Work out the finished part from the listing and answer in its coordinate system (mm). Coordinates: 2 decimals unless noted, no trailing zeros. Order: outer loops, then holes, each group sorted by start corner. A loop starts at its lowest first (then second) coordinate and runs counter-clockwise, first axis right, second up. Notation, with made-up numbers: (73, 84.5) -> (89, 84.5) arc R11 cw to (89, 102.5) -> close; hole circle Ø9 at (78, 89). An arc over 180 degrees is marked (long way). Write item = value, one per line. Start each with the question number.
Q1. Flat-ended cylindrical pins translate along their axes: pin 1 (5 mm diameter, centred on y = -5.5, z = 4.5, fed in from -X); pin 2 (4 mm diameter, centred on y = -13, z = -6.5, fed in from +X); pin 3 (3 mm diameter, centred on y = -15.5, z = -6, fed in from +X). Find the tip coordinate at first contact, or state that the pin passes through.
Q2. The part is cut by section D-D, the plane y = -16.25. Determine the outline of the cut face in (x, z).
Q3. The part is cut by section A-A, the plane x = 0. Determine the outline of the cut face in (y, z) (3 decimals), plus the area to 3 significant figures.
Q4. The part is cut by section C-C, the plane y = -3. Determine the outline of the cut face in (x, z), plus the area to 3 significant figures.
Q5. Straight lines are drawn through the part: L1, parallel to Z at x = 0, y = -1.75; L2, parallel to Z at x = -4.5, y = -5; L3, parallel to X at y = -4.5, z = 2.5. For each, find the intervals that lie inside material, in ascending order. Write a range as from..to.
Q6. The part is cut by section B-B, the plane z = 0. Determine the outline of the cut face in (x, y) (3 decimals).
Q7. For a pull along X with two mould halves and no side action, classify faces 1 (the cylindrical face through (-6.93, -6.72, -5.31)), 2 (the flat face through (7.2, 0, 1.3)), 3 (the cylindrical face through (-1.38, -4.02, -6.2)) as +X half, -X half, draft (parallel to the pull), parting line (faces both ways), or undercut.
```python
from build123d import *

# Parameters (mm, degrees)
CHAMFER1_SIZE = 0.762


with BuildPart() as part:
    # Sketch1 → Revolve1 (revolve)
    with BuildSketch(Plane.XY):
        with BuildLine():
            Line((6.35, 0), (8.73125, 0))
            Line((8.73125, 0), (8.73125, -13.25435082))
            ThreePointArc((8.73125, -13.25435082), (8.567676279, -13.87782567), (8.11909112, -14.340695636))
            Line((8.11909112, -14.340695636), (0.635, -18.872721569))
            ThreePointArc((0.635, -18.872721569), (0.329640957, -19.004848916), (0, -19.05))
            Line((0, -19.05), (0, -13.716))
            ThreePointArc((0, -13.716), (4.490128061, -11.856128061), (6.35, -7.366))
            Line((6.35, -7.366), (6.35, 0))
        make_face()
    revolve(axis=Axis((0, -13.716, 0), (0, -1, 0)))

    # Chamfer1
    chamfer1_edges = [part.edges().sort_by_distance(p)[0] for p in [
        (-6.35, 0, 0),
    ]]
    chamfer(chamfer1_edges, length=CHAMFER1_SIZE)


solid = part.part
```
Model answer:
q1.pin_1 = -8.5
q1.pin_2 = 7.48
q1.pin_3 = 6.44
q2.outline = circle Ø9.93 at (0, 0)
q3.outline = (-18.873, -0.635) -> (-14.341, -8.119) arc R1.27 ccw to (-13.254, -8.731) -> (0, -8.731) -> (0, -7.112) -> (-0.762, -6.35) -> (-7.366, -6.35) arc R6.35 cw to (-7.366, 6.35) -> (-0.762, 6.35) -> (0, 7.112) -> (0, 8.731) -> (-13.254, 8.731) arc R1.27 ccw to (-14.341, 8.119) -> (-18.873, 0.635) arc R1.226 ccw to start
q3.area = 132 mm2
q4.outline = circle Ø17.46 at (0, 0); hole circle Ø12.7 at (0, 0)
q4.area = 113 mm2
q5.L1 = -8.73..-6.35, 6.35..8.73
q5.L2 = -7.48..-4.48, 4.48..7.48
q5.L3 = -8.37..-5.84, 5.84..8.37
q6.outline = (-8.731, -13.254) arc R1.27 ccw to (-8.119, -14.341) -> (-0.635, -18.873) arc R1.226 ccw to (0.635, -18.873) -> (8.119, -14.341) arc R1.27 ccw to (8.731, -13.254) -> (8.731, 0) -> (7.112, 0) -> (6.35, -0.762) -> (6.35, -7.366) arc R6.35 cw to (-6.35, -7.366) -> (-6.35, -0.762) -> (-7.112, 0) -> (-8.731, 0) -> close
q7.face_1 = parting line
q7.face_2 = draft
q7.face_3 = undercut
